```python
from build123d import *

# Parameters (mm, degrees)
SKETCH2_W               = 235.89
SKETCH2_H               = 111.89
BOSS_EXTRUDE1_DEPTH     = 2.5
SKETCH3_R               = 1.25
CUT_EXTRUDE1_DEPTH      = 131.56460489
CUT_EXTRUDE2_DEPTH      = 131.56460489
CUT_EXTRUDE2_DEPTH_BACK = 131.56460489
SKETCH4_R               = 13.1
SKETCH4_R_2             = 18.65
SKETCH4_W               = 45.9288
SKETCH4_H               = 75.4987


with BuildPart() as part:
    # Sketch2 → Boss-Extrude1 (new body)
    with BuildSketch(Plane(origin=(0, 0, 0), x_dir=(1, 0, 0), z_dir=(0, 1, 0))):
        Rectangle(SKETCH2_W, SKETCH2_H)
    extrude(amount=BOSS_EXTRUDE1_DEPTH)

    # Sketch3 → Cut-Extrude1 (cut, through all)
    with BuildSketch(Plane(origin=(0, 2.5, 0), x_dir=(1, 0, 0), z_dir=(0, 1, 0))):
        with Locations(Location((-113.945, 51.945, 0), (0, 0, 270))):
            Circle(SKETCH3_R)
        with Locations(Location((-113.945, -51.945, 0), (0, 0, 270))):
            Circle(SKETCH3_R)
        with Locations(Location((113.945, -51.945, 0), (0, 0, 270))):
            Circle(SKETCH3_R)
        with Locations(Location((113.945, 51.945, 0), (0, 0, 270))):
            Circle(SKETCH3_R)
    extrude(amount=-CUT_EXTRUDE1_DEPTH, mode=Mode.SUBTRACT)

    # Sketch4 → Cut-Extrude2 (cut, two sides: drawn at the far end of the back side and taken through both)
    with BuildSketch(Plane(origin=(0, 2.5, 0), x_dir=(1, 0, 0), z_dir=(0, 1, 0)).offset(-CUT_EXTRUDE2_DEPTH_BACK)):
        with Locations(Location((40.845, 30.6237, 0), (0, 0, 270))):
            Circle(SKETCH4_R)
        with Locations(Location((4.445, 30.6237, 0), (0, 0, 270))):
            Circle(SKETCH4_R)
        with Locations(Location((4.445, -3.7763, 0), (0, 0, 270))):
            Circle(SKETCH4_R_2)
        with Locations((90.3227, 3.89565)):
            Rectangle(SKETCH4_W, SKETCH4_H)
    extrude(amount=CUT_EXTRUDE2_DEPTH + CUT_EXTRUDE2_DEPTH_BACK, mode=Mode.SUBTRACT)


solid = part.part
```
For this review, take the finished solid that the model builds, in its own axes (mm). Round coordinates to 2 decimals unless told otherwise and drop trailing zeros. Write each loop counter-clockwise with the first axis right and the second up, starting at its lowest first coordinate (ties: lowest second). Pieces come first, ordered by that corner, then holes. Notation, with made-up numbers: (64, 44.25) - (78, 44.25) arc R9 cw to (78, 50.25) - close; hole circle Ø8 at (-1.75, -33). An arc over 180 degrees is marked (long way). Answer as CSV lines item,"result". Start each with the question number.
(1) Add section C-C, the plane y = 1. State how many separate pieces and enclosed holes the cut face has, plus the area to 3 significant figures.
(2) Add section D-D, the plane z = -25.5. State the section outline as (x, y) points (3 decimals), plus the area to 3 significant figures.
(3) Add section A-A, the plane x = 99.5. State the section outline as (y, z) points (3 decimals), plus the area to 3 significant figures.
(4) Add section B-B, the plane z = 30. State the section outline as (x, y) points (3 decimals), plus the area to 3 significant figures.
(5) Mouldability with a two-part tool opening along Z and no side actions: class faces 1 (the flat face through (-28, 2.5, -1)), 2 (the cylindrical face through (44.78, 1.23, -18.13)) as +Z half, -Z half, draft (parallel to the pull), parting line (faces both ways), or undercut.
(6) For line 1 (X direction, y = 1.55, z = -31) (3 decimals); line 2 (X direction, y = 2.35, z = 12.5) (3 decimals); line 3 (Z direction, x = -6.5, y = 0.45) (3 decimals), list the stretches that pass through material, from the lowest coordinate up.
From the geometry:
1,separate pieces,"1"
1,enclosed holes,"8"
1,area,"20,700 mm²"
2,outline,"(-117.945, 0) - (-7.611, 0) - (-7.611, 2.5) - (-117.945, 2.5) - close; (16.501, 0) - (28.789, 0) - (28.789, 2.5) - (16.501, 2.5) - close; (52.901, 0) - (67.358, 0) - (67.358, 2.5) - (52.901, 2.5) - close; (113.287, 0) - (117.945, 0) - (117.945, 2.5) - (113.287, 2.5) - close"
2,area,"354 mm²"
3,outline,"(0, -55.945) - (2.5, -55.945) - (2.5, -41.645) - (0, -41.645) - close; (0, 33.854) - (2.5, 33.854) - (2.5, 55.945) - (0, 55.945) - close"
3,area,"91.0 mm²"
4,outline,"(-117.945, 0) - (67.358, 0) - (67.358, 2.5) - (-117.945, 2.5) - close; (113.287, 0) - (117.945, 0) - (117.945, 2.5) - (113.287, 2.5) - close"
4,area,"475 mm²"
5,face 1,"draft"
5,face 2,"undercut"
6,line 1,"x = -117.945 to -8.65, 17.54 to 27.75, 53.94 to 67.358, 113.287 to 117.945"
6,line 2,"x = -117.945 to -12.039, 20.929 to 67.358, 113.287 to 117.945"
6,line 3,"z = -55.945 to -37.822, -23.425 to -11.324, 18.877 to 55.945"
